```python
from build123d import *

# Parameters (mm, degrees)
SKETCH2_R           = 9.525
SKETCH2_R_2         = 6.35
BOSS_EXTRUDE1_DEPTH = 14.699996
BOSS_EXTRUDE2_DEPTH = 9.3000068
SKETCH4_R           = 6.35
CUT_EXTRUDE1_DEPTH  = 2540
SKETCH5_R           = 3.175
CUT_EXTRUDE2_DEPTH  = 2540
SKETCH6_R           = 28
SKETCH6_R_2         = 7.320365212
BOSS_EXTRUDE3_DEPTH = 8.200009
SKETCH8_R           = 19.05
CUT_EXTRUDE3_DEPTH  = 8.200009


with BuildPart() as part:
    # Sketch2 → Boss-Extrude1 (new body)
    with BuildSketch(Plane(origin=(0, 0, 0), x_dir=(1, 0, 0), z_dir=(0, 1, 0))):
        Circle(SKETCH2_R)
        Circle(SKETCH2_R_2, mode=Mode.SUBTRACT)
    extrude(amount=BOSS_EXTRUDE1_DEPTH)

    # Sketch3 → Boss-Extrude2 (add)
    with BuildSketch(Plane.XZ):
        with BuildLine():
            Line((-31.75, -12.7), (-8.058170349, -24.768612943))
            ThreePointArc((-8.058170349, -24.768612943), (5, -28), (18.058170349, -24.768612943))
            Line((18.058170349, -24.768612943), (41.75, -12.7))
            ThreePointArc((41.75, -12.7), (47.023813104, 5.291562459), (31.75, 16.164467204))
            Line((31.75, 16.164467204), (18.058170349, 24.768612943))
            ThreePointArc((18.058170349, 24.768612943), (5, 28), (-8.058170349, 24.768612943))
            Line((-8.058170349, 24.768612943), (-31.75, 12.7))
            ThreePointArc((-31.75, 12.7), (-44.45, 0), (-31.75, -12.7))
        make_face()
    extrude(amount=BOSS_EXTRUDE2_DEPTH)

    # Sketch4 → Cut-Extrude1 (cut)
    with BuildSketch(Plane(origin=(0, 0, 0), x_dir=(1, 0, 0), z_dir=(0, 1, 0))):
        Circle(SKETCH4_R)
    extrude(amount=-CUT_EXTRUDE1_DEPTH, mode=Mode.SUBTRACT)

    # Sketch5 → Cut-Extrude2 (cut)
    with BuildSketch(Plane(origin=(0, 0, 0), x_dir=(1, 0, 0), z_dir=(0, 1, 0))):
        with Locations((-31.75, 0)):
            Circle(SKETCH5_R)
        with Locations((31.75, 0)):
            Circle(SKETCH5_R)
    extrude(amount=-CUT_EXTRUDE2_DEPTH, mode=Mode.SUBTRACT)

    # Sketch6 → Boss-Extrude3 (add)
    with BuildSketch(Plane(origin=(0, 0, 0), x_dir=(1, 0, 0), z_dir=(0, 1, 0))):
        Circle(SKETCH6_R)
        Circle(SKETCH6_R_2, mode=Mode.SUBTRACT)
    extrude(amount=BOSS_EXTRUDE3_DEPTH)

    # Sketch8 → Cut-Extrude3 (cut)
    with BuildSketch(Plane(origin=(0, 8.200009, 0), x_dir=(1, 0, 0), z_dir=(0, 1, 0))):
        with Locations((-31.75, 0)):
            Circle(SKETCH8_R)
        with Locations((31.75, 0)):
            Circle(SKETCH8_R)
    extrude(amount=-CUT_EXTRUDE3_DEPTH, mode=Mode.SUBTRACT)


solid = part.part
```
Design review of the part built by this model. Coordinates are the model's own, in mm. A direction names the side the tool comes from. Coordinates: 2 decimals unless noted, no trailing zeros. Loops run counter-clockwise (first coordinate to the right, second up) from the corner with the lowest first, then second, coordinate; pieces in that order, holes last.
Q1. We need section C-C on x = -1.5. State the section outline as (y, z) points.
Reported:
outline: (-9.3, -27.24) - (0, -27.24) - (0, -27.96) - (8.2, -27.96) - (8.2, -9.41) - (14.7, -9.41) - (14.7, -6.17) - (-9.3, -6.17) - close; (-9.3, 6.17) - (14.7, 6.17) - (14.7, 9.41) - (8.2, 9.41) - (8.2, 27.96) - (0, 27.96) - (0, 27.24) - (-9.3, 27.24) - close
Q2. We need section A-A on z = 0. State the section outline as (x, y) points (3 decimals), and give its area (3 significant figures).
Reported:
outline: (-44.45, -9.3) - (-34.925, -9.3) - (-34.925, 0) - (-44.45, 0) - close; (-28.575, -9.3) - (-6.35, -9.3) - (-6.35, 14.7) - (-9.525, 14.7) - (-9.525, 8.2) - (-12.7, 8.2) - (-12.7, 0) - (-28.575, 0) - close; (6.35, -9.3) - (28.575, -9.3) - (28.575, 0) - (12.7, 0) - (12.7, 8.2) - (9.525, 8.2) - (9.525, 14.7) - (6.35, 14.7) - close; (34.925, -9.3) - (47.914, -9.3) - (47.914, 0) - (34.925, 0) - close
area: 768 mm2
Q3. We need section B-B on y = -4.25. State the section outline as (x, z) points (3 decimals).
Reported:
outline: (-31.75, -12.7) - (-8.058, -24.769) arc R28 ccw to (18.058, -24.769) - (41.75, -12.7) arc R16.164 ccw to (31.75, 16.164) - (18.058, 24.769) arc R28 ccw to (-8.058, 24.769) - (-31.75, 12.7) arc R12.7 ccw to start; hole circle Ø6.35 at (-31.75, 0); hole circle Ø12.7 at (0, 0); hole circle Ø6.35 at (31.75, 0)
Q4. To check wall thickness, follow line 1 (Z direction, x = 0, y = 6.75); line 2 (Z direction, x = -31.75, y = -2.25) (3 decimals); line 3 (Y direction, x = -20, z = 7.5). State the ranges of each line that lie inside material, in increasing order.
Reported:
line 1: z = -28 to -6.35, 6.35 to 28
line 2: z = -12.7 to -3.175, 3.175 to 12.7
line 3: y = -9.3 to 0
Q5. Tool access review of faces 5 (the face through (5, -5, 28)), 6 (the face through (-19.74, -4.58, 18.82)), 7 (the face through (-7.559, 11.405, 5.796)), 8 (the face through (-11, 0, -24)): name each direction out of +Z, -Z, +X, -X, +Y, -Y from which nothing blocks a thin tool from reaching the whole face with its end or side.
Reported:
face 5: +Z, -Y
face 6: +Z, -X, -Y
face 7: +Y
face 8: -Z, -X, -Y
Q6. For pin 1 (1 mm diameter, centred on x = 20.5, y = -3.5, fed in from +Z); pin 2 (22.5 mm diameter, centred on x = 34, z = -7.5, fed in from +Y); pin 3 (8 mm diameter, centred on y = 10, z = 15, fed in from -X); pin 4 (5 mm diameter, centred on x = 19, y = 12, fed in from -Z), all flat-tipped, find the tip position at first contact; note any pin that passes through.
Reported:
pin 1: stops at z = 23.55
pin 2: stops at y = 0
pin 3: stops at x = -22.51
pin 4: passes through
Q7. We need section D-D on y = 5.25. State the section outline as (x, z) points.
Reported:
outline: (-22.51, -16.66) arc R28 ccw to (22.51, -16.66) arc R19.05 cw to (22.51, 16.66) arc R28 ccw to (-22.51, 16.66) arc R19.05 cw to start; hole circle Ø12.7 at (0, 0)
Q8. The part is to be moulded in two halves that separate along X. For faces 1 (the face through (25, 0, 0)), 2 (the face through (-34.92, -4.58, -0.14)), 3 (the face through (29.74, -4.58, -18.82)), 4 (the face through (-20.07, -4.58, -18.65)), say which applies: +X half, -X half, draft (parallel to the pull), parting line (faces both ways), or undercut.
Reported:
face 1: draft
face 2: undercut
face 3: +X half
face 4: -X half
